Design review of the part built by this model. Coordinates are the model's own, in mm. A direction names the side the tool comes from. Coordinates: 2 decimals unless noted, no trailing zeros. Order: outer loops, then holes, each group sorted by start corner. A loop starts at its lowest first (then second) coordinate and runs counter-clockwise, first axis right, second up. Notation, with made-up numbers: (42.5, 9.25) -> (61.5, 9.25) arc R25 cw to (61.5, 35.25) -> close; hole circle Ø2 at (-21.75, 55). An arc over 180 degrees is marked (long way). Write item = value, one per line.
```python
from build123d import *

# Parameters (mm, degrees)
CROQUIS1_W              = 40
CROQUIS1_H              = 47
CROQUIS1_W_2            = 15
CROQUIS1_H_2            = 41
SALIENTE_EXTRUIR1_DEPTH = 3
CROQUIS3_W              = 40
CROQUIS3_H              = 3
SALIENTE_EXTRUIR2_DEPTH = 5
SALIENTE_EXTRUIR3_DEPTH = 3
CROQUIS6_W              = 40
CROQUIS6_H              = 3
SALIENTE_EXTRUIR4_DEPTH = 8.5
CROQUIS7_W              = 11.5
CROQUIS7_H              = 3
SALIENTE_EXTRUIR5_DEPTH = 15
CROQUIS8_W              = 64.003791446
CROQUIS8_H              = 3
SALIENTE_EXTRUIR7_DEPTH = 53
CROQUIS9_W              = 24.723137679
CROQUIS9_H              = 41
CROQUIS9_W_2            = 12.312971116
CORTAR_EXTRUIR1_DEPTH   = 53


with BuildPart() as part:
    # Croquis1 → Saliente-Extruir1 (new body)
    with BuildSketch(Plane(origin=(0, 0, 0), x_dir=(1, 0, 0), z_dir=(0, 1, 0))):
        Rectangle(CROQUIS1_W, CROQUIS1_H)
        with Locations((-9.5, 0)):
            Rectangle(CROQUIS1_W_2, CROQUIS1_H_2, mode=Mode.SUBTRACT)
        with Locations((9.5, 0)):
            Rectangle(CROQUIS1_W_2, CROQUIS1_H_2, mode=Mode.SUBTRACT)
    extrude(amount=SALIENTE_EXTRUIR1_DEPTH)

    # Croquis3 → Saliente-Extruir2 (add)
    with BuildSketch(Plane(origin=(0, 3, 0), x_dir=(1, 0, 0), z_dir=(0, 1, 0))):
        with Locations((0, 22)):
            Rectangle(CROQUIS3_W, CROQUIS3_H)
        with Locations((0, -22)):
            Rectangle(CROQUIS3_W, CROQUIS3_H)
    extrude(amount=SALIENTE_EXTRUIR2_DEPTH)

    # Croquis5 → Saliente-Extruir3 (add)
    with BuildSketch(Plane.XY.offset(-20.5)):
        with BuildLine():
            Line((-10.5, 6.5), (-2.5, 6.5))
            ThreePointArc((-2.5, 6.5), (-2.146446609, 6.646446609), (-2, 7))
            Line((-2, 7), (-2, 8))
            Line((-2, 8), (-11, 8))
            Line((-11, 8), (-11, 7))
            ThreePointArc((-11, 7), (-10.853553391, 6.646446609), (-10.5, 6.5))
        make_face()
        with BuildLine():
            Line((2, 7), (2, 8))
            Line((2, 8), (11, 8))
            Line((11, 8), (11, 7))
            ThreePointArc((11, 7), (10.853553391, 6.646446609), (10.5, 6.5))
            Line((10.5, 6.5), (2.5, 6.5))
            ThreePointArc((2.5, 6.5), (2.146446609, 6.646446609), (2, 7))
        make_face()
    saliente_extruir3 = extrude(amount=SALIENTE_EXTRUIR3_DEPTH)

    # Simetría3: Saliente-Extruir3 across plane
    add(saliente_extruir3.mirror(Plane.XY))

    # Croquis6 → Saliente-Extruir4 (add)
    with BuildSketch(Plane.XY.offset(23.5)):
        with Locations((0, 1.5)):
            Rectangle(CROQUIS6_W, CROQUIS6_H)
    saliente_extruir4 = extrude(amount=SALIENTE_EXTRUIR4_DEPTH)

    # Simetría4: Saliente-Extruir4 across plane
    add(saliente_extruir4.mirror(Plane.XY))

    # Croquis7 → Saliente-Extruir5 (add)
    with BuildSketch(Plane.ZY.offset(20)):
        with Locations((-26.25, 1.5)):
            Rectangle(CROQUIS7_W, CROQUIS7_H)
        with Locations((26.25, 1.5)):
            Rectangle(CROQUIS7_W, CROQUIS7_H)
    extrude(amount=SALIENTE_EXTRUIR5_DEPTH)

    # Croquis8 → Saliente-Extruir7 (add)
    with BuildSketch(Plane(origin=(20, 0, 0), x_dir=(0, 0, -1), z_dir=(1, 0, 0))):
        with Locations((0.001895723, 1.5)):
            Rectangle(CROQUIS8_W, CROQUIS8_H)
    extrude(amount=SALIENTE_EXTRUIR7_DEPTH)

    # Croquis9 → Cortar-Extruir1 (cut)
    with BuildSketch(Plane(origin=(0, 3, 0), x_dir=(1, 0, 0), z_dir=(0, 1, 0))):
        with Locations((32.36156884, 0)):
            Rectangle(CROQUIS9_W, CROQUIS9_H)
        with Locations((58.925723175, 0)):
            Rectangle(CROQUIS9_W_2, CROQUIS9_H)
    extrude(amount=-CORTAR_EXTRUIR1_DEPTH, mode=Mode.SUBTRACT)


solid = part.part
```
(1) Insertion check: pin 1 (0.5 mm diameter, centred on y = 7.5, z = -19, fed in from -X); pin 2 (0.9 mm diameter, centred on x = 8, z = -19, fed in from -Y); pin 3 (2.5 mm diameter, centred on y = 6.5, z = -21.5, fed in from -X); pin 4 (2 mm diameter, centred on y = 4.5, z = 1, fed in from +X). Each pin has a flat end and moves straight along its axis. Give the tip position at first contact, or say it passes through.
Report:
pin_1 = -11
pin_2 = 6.5
pin_3 = -20
pin_4 = through
(2) We need section B-B (x = 35). Write out the cut boundary in (y, z), and give its area (3 significant figures).
Report:
outline = (0, -32) -> (3, -32) -> (3, -20.5) -> (0, -20.5) -> close; (0, 20.5) -> (3, 20.5) -> (3, 32) -> (0, 32) -> close
area = 69.0 mm²
(3) We need section C-C (y = 4.25). Write out the cut boundary in (x, z).
Report:
outline = (-20, -23.5) -> (20, -23.5) -> (20, -20.5) -> (-20, -20.5) -> close; (-20, 20.5) -> (20, 20.5) -> (20, 23.5) -> (-20, 23.5) -> close
(4) The part is to be moulded in two halves that separate along X. For faces 1 (the flat face through (0, 3, 0)), 2 (the flat face through (32, 2, 20.5)), 3 (the flat face through (-35, 2, 26)), say which applies: released by +X, released by -X, zero draft, split by the parting line, or undercut.
Report:
face_1 = zero draft
face_2 = undercut
face_3 = released by -X
(5) For L1, parallel to Z at x = -4, y = 0.5; L2, parallel to Z at x = -5, y = 5.5; L3, parallel to Y at x = 50, z = 3.5, list the stretches that pass through material, from the lowest coordinate up.
Report:
L1 = -32 to -20.5, 20.5 to 32
L2 = -23.5 to -20.5, 20.5 to 23.5
L3 = 0 to 3
(6) We need section A-A (z = -4). Write out the cut boundary in (x, y), and give its area (3 significant figures).
Report:
outline = (-20, 0) -> (-17, 0) -> (-17, 3) -> (-20, 3) -> close; (-2, 0) -> (2, 0) -> (2, 3) -> (-2, 3) -> close; (17, 0) -> (20, 0) -> (20, 3) -> (17, 3) -> close; (44.72, 0) -> (52.77, 0) -> (52.77, 3) -> (44.72, 3) -> close; (65.08, 0) -> (73, 0) -> (73, 3) -> (65.08, 3) -> close
area = 77.9 mm²
(7) For faces 4 (the flat face through (52.769, 2, 0)), 5 (the flat face through (2, 1, 0)), 6 (the flat face through (-7, 6.5, -19)), list the 3-axis set-ups (+Z, -Z, +X, -X, +Y, -Y) from which the entire face can be reached by the end or side of a thin tool; tool diameter is ignored.
Report:
face_4 = +Y, -Y
face_5 = -Y
face_6 = +X, -X, -Y
